The model under review builds one solid part; all positions refer to its coordinate system, in mm. Give positions to 0.01 mm unless a question says otherwise; leave off trailing zeros. Order: outer loops, then holes, each group sorted by start corner. A loop starts at its lowest first (then second) coordinate and runs counter-clockwise, first axis right, second up. Notation, with made-up numbers: (68.25, -16) - (119.25, -16) arc R22 ccw to (119.25, 10) - close; hole circle Ø5 at (71, 8). An arc over 180 degrees is marked (long way). Use CSV: the item, a comma, the result in double quotes. Start each with the question number.
```python
from build123d import *

# Parameters (mm, degrees)
SKETCH_1_W          = 450
SKETCH_1_H          = 390
SKETCH_1_R          = 82.5
EXTRUDE_1_DEPTH     = 24
CUT_EXTRUDE_START   = 24
SKETCH_1_3_R        = 4
SKETCH_1_3_R_2      = 7
CUT_EXTRUDE_1_DEPTH = 18


with BuildPart() as part:
    # 草图1 → 凸台-拉伸1 (new body)
    with BuildSketch(Plane.XY):
        Rectangle(SKETCH_1_W, SKETCH_1_H)
        with Locations((-45, 0)):
            Circle(SKETCH_1_R, mode=Mode.SUBTRACT)
    extrude(amount=EXTRUDE_1_DEPTH)

    # 草图1<3> → 切除-拉伸1 (cut)
    with BuildSketch(Plane.XY.offset(CUT_EXTRUDE_START)):
        with Locations(Location((-45, 92.5, 0), (0, 0, 180))):
            Circle(SKETCH_1_3_R)
        with Locations(Location((9.370135837, 74.83407198, 0), (0, 0, 180))):
            Circle(SKETCH_1_3_R)
        with Locations(Location((42.972727757, 28.58407198, 0), (0, 0, 180))):
            Circle(SKETCH_1_3_R)
        with Locations(Location((42.972727757, -28.58407198, 0), (0, 0, 180))):
            Circle(SKETCH_1_3_R)
        with Locations(Location((9.370135837, -74.83407198, 0), (0, 0, 180))):
            Circle(SKETCH_1_3_R)
        with Locations(Location((-45, -92.5, 0), (0, 0, 180))):
            Circle(SKETCH_1_3_R)
        with Locations(Location((-99.370135837, -74.83407198, 0), (0, 0, 180))):
            Circle(SKETCH_1_3_R)
        with Locations(Location((-132.972727757, -28.58407198, 0), (0, 0, 180))):
            Circle(SKETCH_1_3_R)
        with Locations(Location((-132.972727757, 28.58407198, 0), (0, 0, 180))):
            Circle(SKETCH_1_3_R)
        with Locations(Location((-99.370135837, 74.83407198, 0), (0, 0, 180))):
            Circle(SKETCH_1_3_R)
        with Locations(Location((0, 180, 0), (0, 0, 180))):
            Circle(SKETCH_1_3_R_2)
        with Locations(Location((-175, 180, 0), (0, 0, 180))):
            Circle(SKETCH_1_3_R_2)
        with Locations(Location((175, 180, 0), (0, 0, 180))):
            Circle(SKETCH_1_3_R_2)
        with Locations(Location((-175, -180, 0), (0, 0, 180))):
            Circle(SKETCH_1_3_R_2)
        with Locations(Location((0, -180, 0), (0, 0, 180))):
            Circle(SKETCH_1_3_R_2)
        with Locations(Location((175, -180, 0), (0, 0, 180))):
            Circle(SKETCH_1_3_R_2)
    extrude(amount=-CUT_EXTRUDE_1_DEPTH, mode=Mode.SUBTRACT)


solid = part.part
```
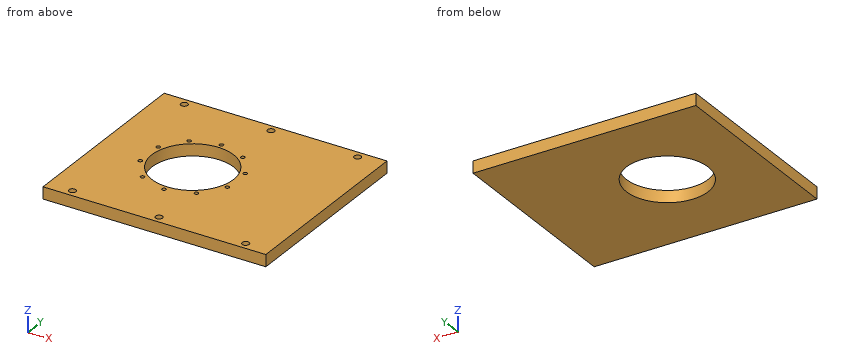
1. To check wall thickness, follow L1, parallel to X at y = 180, z = 15.25; L2, parallel to X at y = 92.5, z = 11; L3, parallel to Y at x = -172, z = 15.5. State the ranges of each line that lie inside material, in increasing order. Write a range as [from, to].
2. Consider section B-B (x = 175). Give the boundary of the cut face in (y, z).
3. Consider section D-D (y = -180). Give the boundary of the cut face in (x, z), and give its area (3 significant figures).
4. Clearance check with a flat-ended pin moving along its axis: pin 1 (12.5 mm diameter, centred on x = 175, y = 180, fed in from +Z). State where the tip first meets the part, or that it passes through.
5. Consider section A-A (y = 0). Give the boundary of the cut face in (x, z).
6. Consider section C-C (x = -88). Give the boundary of the cut face in (y, z).
Answers follow:
1,L1,"x = [-225, -182], [-168, -7], [7, 168], [182, 225]"
1,L2,"x = [-225, -49], [-41, 225]"
1,L3,"y = [-195, -186.32], [-173.68, 173.68], [186.32, 195]"
2,outline,"(-195, 0) - (195, 0) - (195, 24) - (187, 24) - (187, 6) - (173, 6) - (173, 24) - (-173, 24) - (-173, 6) - (-187, 6) - (-187, 24) - (-195, 24) - close"
3,outline,"(-225, 0) - (225, 0) - (225, 24) - (182, 24) - (182, 6) - (168, 6) - (168, 24) - (7, 24) - (7, 6) - (-7, 6) - (-7, 24) - (-168, 24) - (-168, 6) - (-182, 6) - (-182, 24) - (-225, 24) - close"
3,area,"10,000 mm^2"
4,pin 1,"stops at z = 6"
5,outline,"(-225, 0) - (-127.5, 0) - (-127.5, 24) - (-225, 24) - close; (37.5, 0) - (225, 0) - (225, 24) - (37.5, 24) - close"
6,outline,"(-195, 0) - (-70.41, 0) - (-70.41, 24) - (-195, 24) - close; (70.41, 0) - (195, 0) - (195, 24) - (70.41, 24) - close"
